Autodesk Inventor part; units mm, degrees
ref_plane "YZ Plane" through (0, 0, 0) normal (1, 0, 0) x (0, 1, 0)
ref_plane "XZ Plane" through (0, 0, 0) normal (0, 1, 0) x (-1, 0, 0)
ref_plane "XY Plane" through (0, 0, 0) normal (0, 0, 1) x (1, 0, 0)
sketch "Sketch1" plane through (0, 0, 0) normal (0, 1, 0) x (-1, 0, 0)
  line L0 (26, -28) -> (-27.5, -28)
  line L1 (-27.5, -28) -> (-27.5, 38.15)
  line L2 (26, 38.15) -> (26, -28)
  line L3 (26, 38.15) -> (23.15, 38.15)
  line L4 (23.15, 38.15) -> (20.59, 40.75)
  line L5 (20.59, 40.75) -> (-12.27, 40.75)
  line L6 (-12.27, 40.75) -> (-14.9, 38.15)
  line L7 (-14.9, 38.15) -> (-27.5, 38.15)
  point P0 (0, 0)
  point P1 (-27.5, 40.75)
  point P2 (26, 40.75)
  point P3 (4.16, 40.75)
  point P4 (24.575, 38.15)
  point P5 (-21.2, 38.15)
  dimension "d2" = 53.5
  dimension "d12" = 68.75
  dimension "d13" = 2.6
  dimension "d14" = 2.85
  dimension "d15" = 2.56
  dimension "d16" = 32.86
  dimension "d17" = 12.6
  dimension "d18" = 28
  dimension "d19" = 26
extrude "Extrusion1" add sketch "Sketch1" along normal blind 1.6
chamfer "Chamfer1" distance 2 angle 45 1 edges at (27.5, 0.8, 38.15)
chamfer "Chamfer2" distance 0.5 angle 45 3 edges at (-26, 0.8, 38.15) (-26, 0.8, -28) (27.5, 0.8, -28)
sketch "Sketch2" plane through (0, 1.6, 0) normal (0, 1, 0) x (1, 0, 0)
  line L0 (-26, 27.5) -> (-26, -37.65)
  line L1 (27, 28) -> (-25.5, 28)
  line L2 (27.5, -36.15) -> (27.5, 27.5)
  line L3 (-20.59, -40.75) -> (12.27, -40.75)
  point P0 (0, 0)
  point P1 (-23.3, 14.21)
  point P2 (25.32, 13)
  point P3 (9.5, -38.37)
  point P4 (-18.52, -38.37)
  dimension "d28" = 2.7
  dimension "d29" = 13.79
  dimension "d30" = 2.18
  dimension "d31" = 15
  dimension "d32" = 7.48
  dimension "d33" = 2.38
  dimension "d34" = 18
hole "Hole1" at (-23.3, 1.6, -14.21) at (25.32, 1.6, -13) at (9.5, 1.6, 38.37) at (-18.52, 1.6, 38.37) direction (0, -1, 0) diameter 3.4 end through all
properties part number "ArduinoUnoFootprintPART"
CAD build for the part. Positions are in the model's coordinates, mm. A direction names the side the tool comes from. Give positions to 0.01 mm unless a question says otherwise; leave off trailing zeros. Loops run counter-clockwise (first coordinate to the right, second up) from the corner with the lowest first, then second, coordinate; pieces in that order, holes last. Notation, with made-up numbers: M 15.5,-22.75 L 70.5,-22.75 A27 ccw 70.5,-2.75 Z; hole C 72.25,12 d10. An arc over 180 degrees is marked long. One line per question, with ' | ' between items. Start each with the question number.
1. Probe L1, parallel to Z at x = 25.32, y = 1; L2, parallel to Z at x = -18.52, y = 1.35; L3, parallel to X at y = 0.3, z = 38.37. List the from-to ranges inside material, lowest first. Write a range as from..to.
2. 3-axis set-ups, long thin cutter, end or side, ignore diameter. For faces 1 (the face through (-18.59, 0.79, 36.67)), 2 (the face through (-24, 1, 38.15)): which of +Z, -Z, +X, -X, +Y, -Y reach the whole face in a straight line?
3. Saw through at A-A on x = -18.52. Give the cut face in (y, z).
4. Two-plate mould, pull along Z, no slides. Class faces 3 (the face through (23.634, 0.789, -13.221)), 4 (the face through (27.5, 1, 4)), 5 (the face through (20, 1, 38.15)), 6 (the face through (0, 1, -28)): pulls with the +Z half, pulls with the -Z half, needs draft (parallel to the pull), parting line crosses it, or undercut.
5. Flat gauge pin, fed straight in: pin 1 (5.5 mm diameter, centred on x = -18.52, z = 38.37, fed in from +Y). Where does the tip first touch, or does it go through?
6. Saw through at B-B on y = 0.6. Give the cut face in (x, z), plus the area to 3 significant figures.
Result sheet:
1) L1: z = -28..-14.7, -11.3..38.15 | L2: z = -28..36.67, 40.07..40.75 | L3: x = -22.93..-20.22, -16.82..7.8, 11.2..14.68
2) face 1: +Y, -Y | face 2: +Z, -X, +Y, -Y
3) outline: M 0,-28 L 1.6,-28 L 1.6,36.67 L 0,36.67 Z; M 0,40.07 L 1.6,40.07 L 1.6,40.75 L 0,40.75 Z
4) face 3: undercut | face 4: needs draft | face 5: pulls with the +Z half | face 6: pulls with the -Z half
5) pin 1: stops at y = 1.6
6) outline: M -26,-27.5 L -25.5,-28 L 27,-28 L 27.5,-27.5 L 27.5,36.15 L 25.5,38.15 L 14.9,38.15 L 12.27,40.75 L -20.59,40.75 L -23.15,38.15 L -25.5,38.15 L -26,37.65 Z; hole C -23.3,-14.21 d3.4; hole C -18.52,38.37 d3.4; hole C 9.5,38.37 d3.4; hole C 25.32,-13 d3.4 | area: 3,590 mm^2
